```python
from build123d import *

# Parameters (mm, degrees)
F0_W      = 76.2
F0_H      = 50.8
F0_R      = 12.7
F1_DEPTH  = 12.7
F2_W      = 6.35
F2_H      = 50.8
F3_DEPTH  = 5.08
F5_DEPTH  = 50.801
F6_R      = 4.7625
F7_DEPTH  = 15.24
F8_R      = 3.4489881571
F9_DEPTH  = 12.701
F10_R     = 4.2111787038
F11_DEPTH = 113


# Not quite as in the source:
# - an extrude ends at something that could not be found from the text; its depth is read off the source's solid


with BuildPart() as f1:
    # F0 (on Top) → F1 (new body)
    with BuildSketch(Plane.XY):
        Rectangle(F0_W, F0_H)
        Circle(F0_R, mode=Mode.SUBTRACT)
    extrude(amount=F1_DEPTH)

    # F2 (on face) → F3 (cut)
    with BuildSketch(Plane.XY.offset(12.7)):
        with Locations((-32.385, 0)):
            Rectangle(F2_W, F2_H)
        with BuildLine():
            Line((6.35, 25.4), (-6.35, 25.4))
            Line((-6.35, 25.4), (-6.35, 10.9985226281))
            ThreePointArc((-6.35, 10.9985226281), (0, 12.7), (6.35, 10.9985226281))
            Line((6.35, 10.9985226281), (6.35, 25.4))
        make_face()
        with BuildLine():
            Line((-6.35, -10.9985226281), (-6.35, -25.4))
            Line((-6.35, -25.4), (6.35, -25.4))
            Line((6.35, -25.4), (6.35, -10.9985226281))
            ThreePointArc((6.35, -10.9985226281), (0, -12.7), (-6.35, -10.9985226281))
        make_face()
    extrude(amount=-F3_DEPTH, mode=Mode.SUBTRACT)

    # F4 (on face) → F5 (cut, through all)
    with BuildSketch(Plane.XZ.offset(25.4)):
        Polygon((31.75, 12.7), (19.05, 12.7), (16.1170606325, 7.62), (34.6829393675, 7.62), align=None)
    extrude(amount=-F5_DEPTH, mode=Mode.SUBTRACT)

    # F6 (on face) → F7 (join)
    with BuildSketch(Plane.YZ.offset(38.1)):
        with Locations((0, 6.35)):
            Circle(F6_R)
    extrude(amount=F7_DEPTH)

    # F8 (on face) → F9 (cut, through all)
    with BuildSketch(Plane.XY.offset(12.7)):
        with Locations((-24.371592328, 2.9855815228)):
            Circle(F8_R)
    extrude(amount=-F9_DEPTH, mode=Mode.SUBTRACT)

    # F10 (on face) → F11 (cut, through all)
    with BuildSketch(Plane.XY.offset(12.7)):
        with Locations((-20.9910459816, -11.7274438962)):
            Circle(F10_R)
    extrude(amount=F11_DEPTH, mode=Mode.SUBTRACT)


solid = f1.part
```
Design review of the part built by this model. Coordinates are the model's own, in mm. A direction names the side the tool comes from. Round coordinates to 2 decimals unless told otherwise and drop trailing zeros. Write each loop counter-clockwise with the first axis right and the second up, starting at its lowest first coordinate (ties: lowest second). Pieces come first, ordered by that corner, then holes. Notation, with made-up numbers: (-23.5, -27.5) -> (10.5, -27.5) arc R5 cw to (10.5, -19.5) -> close; hole circle Ø11 at (-6, 67). An arc over 180 degrees is marked (long way). Write item = value, one per line. Start each with the question number.
1) Mouldability with a two-part tool opening along Z and no side actions: class faces 3 (the face through (-35.56, 0, 10)), 4 (the face through (17.604, -0.356, 10.196)), 5 (the face through (14, 0, 12.7)) as +Z half, -Z half, draft (parallel to the pull), parting line (faces both ways), or undercut.
2) Wall thickness on probe 1 along Y at (x, z) = (-0.5, 6.5); probe 2 along X at (y, z) = (21, 10); probe 3 along Y at (x, z) = (-11, 4.25): over which ranges is each line inside the solid? List them lowest first. Write a range as from..to.
3) Take a section at C-C, the plane y = -9. State the section outline as (x, z) points.
4) Take a section at A-A, the plane x = 0. State the section outline as (y, z) points.
5) Tool access review of faces 1 (the face through (-29.21, 0, 10)), 2 (the face through (-1.653, 12.592, 6.261)): name each direction out of +Z, -Z, +X, -X, +Y, -Y from which nothing blocks a thin tool from reaching the whole face with its end or side.
6) Take a section at D-D, the plane y = -14.5. State the section outline as (x, z) points, plus the area to 3 significant figures.
7) Take a section at B-B, the plane z = 6.35. State the section outline as (x, y) points.
8) Clearance check with flat-ended pins moving along their axes: pin 1 (3 mm diameter, centred on y = 13, z = 3.5, fed in from +X); pin 2 (4 mm diameter, centred on x = -1, y = 19.5, fed in from +Z). State where each tip first meets the part, or that it passes through.
Results list:
q1.face_3 = draft
q1.face_4 = undercut
q1.face_5 = +Z half
q2.probe_1 = -25.4..-12.69, 12.69..25.4
q2.probe_2 = -38.1..-35.56, -29.21..-6.35, 6.35..17.49, 33.31..38.1
q2.probe_3 = -25.4..-6.35, 6.35..25.4
q3.outline = (-38.1, 0) -> (-8.96, 0) -> (-8.96, 12.7) -> (-29.21, 12.7) -> (-29.21, 7.62) -> (-35.56, 7.62) -> (-35.56, 12.7) -> (-38.1, 12.7) -> close; (8.96, 0) -> (38.1, 0) -> (38.1, 12.7) -> (31.75, 12.7) -> (34.68, 7.62) -> (16.12, 7.62) -> (19.05, 12.7) -> (8.96, 12.7) -> close
q4.outline = (-25.4, 0) -> (-12.7, 0) -> (-12.7, 7.62) -> (-25.4, 7.62) -> close; (12.7, 0) -> (25.4, 0) -> (25.4, 7.62) -> (12.7, 7.62) -> close
q5.face_1 = +Z, +Y, -Y
q5.face_2 = +Z, -Z
q6.outline = (-38.1, 0) -> (38.1, 0) -> (38.1, 12.7) -> (31.75, 12.7) -> (34.68, 7.62) -> (16.12, 7.62) -> (19.05, 12.7) -> (6.35, 12.7) -> (6.35, 7.62) -> (-6.35, 7.62) -> (-6.35, 12.7) -> (-29.21, 12.7) -> (-29.21, 7.62) -> (-35.56, 7.62) -> (-35.56, 12.7) -> (-38.1, 12.7) -> close
q6.area = 792 mm²
q7.outline = (-38.1, -25.4) -> (38.1, -25.4) -> (38.1, -4.76) -> (53.34, -4.76) -> (53.34, 4.76) -> (38.1, 4.76) -> (38.1, 25.4) -> (-38.1, 25.4) -> close; hole circle Ø6.9 at (-24.37, 2.99); hole circle Ø25.4 at (0, 0)
q8.pin_1 = 38.1
q8.pin_2 = 7.62
